Verification items for the finished model (mm, model axes). Face numbers are marked on the shaded views. A direction names the side the tool comes from. Coordinates: 2 decimals unless noted, no trailing zeros. Order: outer loops, then holes, each group sorted by start corner. A loop starts at its lowest first (then second) coordinate and runs counter-clockwise, first axis right, second up.
Q1. Cross-section at C-C, the plane y = 8.5. Record the boundary of the cut face in (x, z), and give its area (3 significant figures).
Q2. Cross-section at A-A, the plane x = 45. Record the boundary of the cut face in (y, z), and give its area (3 significant figures).
Q3. Set-up check for the marked faces 1 and 2: record each of +Z, -Z, +X, -X, +Y, -Y from which the full face is reachable in a straight line by a thin tool's end or side.
Q4. Cross-section at D-D, the plane z = 35. Record the boundary of the cut face in (x, y).
Q5. Depth check by flat-ended pin: P1, Ø8, axis at x = 26.75, z = 8, coming from the +Y side; P2, Ø2.5, axis at x = 37, y = 17, coming from the +Z side. Enter the tip coordinate at first touch or a pass-through.
Q6. Draft check along X on the marked faces 3, 4, 5 and 6. Enter one of: pulls with the +X half, pulls with the -X half, needs draft (parallel to the pull), parting line crosses it, or undercut.
Q7. Thickness scan on line 1 (X direction, y = 21, z = 39); line 2 (Y direction, x = 45, z = 10); line 3 (Y direction, x = 45, z = 31.5). Record the ranges inside material, lowest first.
Q8. Cross-section at B-B, the plane x = 26.75. Record the boundary of the cut face in (y, z).
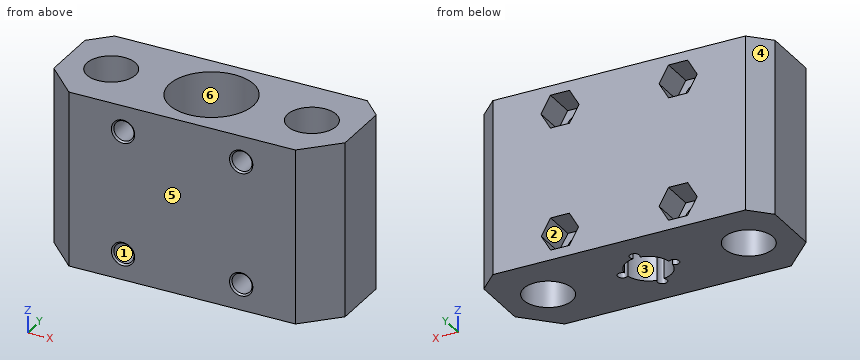
from build123d import *

# Parameters (mm, degrees)
SKETCH1_W           = 90
SKETCH1_H           = 34
SKETCH1_R           = 7
SKETCH1_R_2         = 7.5
BOSS_EXTRUDE1_DEPTH = 54
CHAMFER1_SIZE       = 6
CHAMFER2_SIZE       = 10
SKETCH2_R           = 13
CUT_EXTRUDE1_DEPTH  = 32
SKETCH3_R           = 3.1
CUT_EXTRUDE2_DEPTH  = 111.326787318
CUT_EXTRUDE3_DEPTH  = 10
SKETCH5_R           = 1.5
CUT_EXTRUDE4_DEPTH  = 102.390334845
CIRPATTERN1_COUNT   = 4
CHAMFER3_SIZE       = 0.5


with BuildPart() as part:
    # Sketch1 → Boss-Extrude1 (new body)
    with BuildSketch(Plane.XY):
        with Locations((45, 17)):
            Rectangle(SKETCH1_W, SKETCH1_H)
        with Locations((45, 17)):
            Circle(SKETCH1_R, mode=Mode.SUBTRACT)
        with Locations((14, 17)):
            Circle(SKETCH1_R_2, mode=Mode.SUBTRACT)
        with Locations((76, 17)):
            Circle(SKETCH1_R_2, mode=Mode.SUBTRACT)
    extrude(amount=BOSS_EXTRUDE1_DEPTH)

    # Chamfer1
    chamfer1_edges = [part.edges().sort_by_distance(p)[0] for p in [
        (0, 34, 27),
        (90, 34, 27),
    ]]
    chamfer(chamfer1_edges, length=CHAMFER1_SIZE)

    # Chamfer2
    chamfer2_edges = [part.edges().sort_by_distance(p)[0] for p in [
        (90, 0, 27),
        (0, 0, 27),
    ]]
    chamfer(chamfer2_edges, length=CHAMFER2_SIZE)

    # Sketch2 → Cut-Extrude1 (cut)
    with BuildSketch(Plane.XY.offset(54)):
        with Locations((45, 17)):
            Circle(SKETCH2_R)
    extrude(amount=-CUT_EXTRUDE1_DEPTH, mode=Mode.SUBTRACT)

    # Sketch3 → Cut-Extrude2 (cut, through all)
    with BuildSketch(Plane(origin=(0, 34, 0), x_dir=(1, 0, 0), z_dir=(0, 1, 0))):
        with Locations(Location((26.75, -8, 0), (0, 0, 270))):
            Circle(SKETCH3_R)
        with Locations(Location((63.25, -8, 0), (0, 0, 270))):
            Circle(SKETCH3_R)
        with Locations(Location((63.25, -46, 0), (0, 0, 270))):
            Circle(SKETCH3_R)
        with Locations(Location((26.75, -46, 0), (0, 0, 270))):
            Circle(SKETCH3_R)
    extrude(amount=-CUT_EXTRUDE2_DEPTH, mode=Mode.SUBTRACT)

    # Sketch4 → Cut-Extrude3 (cut)
    with BuildSketch(Plane(origin=(0, 34, 0), x_dir=(1, 0, 0), z_dir=(0, 1, 0))):
        Polygon((23.805513627, -13.1), (29.694486373, -13.1), (32.638972746, -8), (29.694486373, -2.9), (23.805513627, -2.9), (20.861027254, -8), align=None)
        Polygon((60.363248654, -13), (66.136751346, -13), (69.023502692, -8), (66.136751346, -3), (60.363248654, -3), (57.476497308, -8), align=None)
        Polygon((60.305513627, -51.1), (66.194486373, -51.1), (69.138972746, -46), (66.194486373, -40.9), (60.305513627, -40.9), (57.361027254, -46), align=None)
        Polygon((29.694486373, -51.1), (32.638972746, -46), (29.694486373, -40.9), (23.805513627, -40.9), (20.861027254, -46), (23.805513627, -51.1), align=None)
    extrude(amount=-CUT_EXTRUDE3_DEPTH, mode=Mode.SUBTRACT)

    # Sketch5 → Cut-Extrude4 (cut, through all)
    with BuildSketch(Plane.XY.offset(22)):
        with Locations((45, 25)):
            Circle(SKETCH5_R)
    cut_extrude4 = extrude(amount=-CUT_EXTRUDE4_DEPTH, mode=Mode.SUBTRACT)

    # CirPattern1: Cut-Extrude4 ×4 about axis
    cirpattern1_axis = Axis((45, 17, 0), (0, 0, 1))
    for i in range(1, CIRPATTERN1_COUNT):
        add(cut_extrude4.rotate(cirpattern1_axis, i * 360 / CIRPATTERN1_COUNT), mode=Mode.SUBTRACT)

    # Chamfer3
    chamfer3_edges = [part.edges().sort_by_distance(p)[0] for p in [
        (26.75, 0, 42.9),
        (63.25, 0, 42.9),
        (63.25, 0, 4.9),
        (26.75, 0, 4.9),
    ]]
    chamfer(chamfer3_edges, length=CHAMFER3_SIZE)


solid = part.part
Check values:
1. outline: (1.5, 0) - (43.59, 0) - (43.59, 22) - (35.16, 22) - (35.16, 54) - (1.5, 54) - close; (46.41, 0) - (88.5, 0) - (88.5, 54) - (54.84, 54) - (54.84, 22) - (46.41, 22) - close; hole circle Ø6.2 at (26.75, 8); hole circle Ø6.2 at (26.75, 46); hole circle Ø6.2 at (63.25, 8); hole circle Ø6.2 at (63.25, 46)
1. area: 3,890 mm2
2. outline: (0, 0) - (7.5, 0) - (7.5, 22) - (4, 22) - (4, 54) - (0, 54) - close; (26.5, 0) - (34, 0) - (34, 54) - (30, 54) - (30, 22) - (26.5, 22) - close
2. area: 586 mm2
3. face 1: +Y, -Y
3. face 2: +Y
4. outline: (0, 10) - (10, 0) - (80, 0) - (90, 10) - (90, 28) - (84, 34) - (6, 34) - (0, 28) - close; hole circle Ø15 at (14, 17); hole circle Ø26 at (45, 17); hole circle Ø15 at (76, 17)
5. P1: stops at y = 24
5. P2: passes through
6. face 3: undercut
6. face 4: pulls with the -X half
6. face 5: needs draft
6. face 6: undercut
7. line 1: x = 0 to 7.66, 20.34 to 32.63, 57.37 to 69.66, 82.34 to 90
7. line 2: y = 0 to 7.5, 26.5 to 34
7. line 3: y = 0 to 4, 30 to 34
8. outline: (0, 0) - (34, 0) - (34, 2.9) - (24, 2.9) - (24, 4.9) - (0.5, 4.9) - (0, 4.4) - close; (0, 11.6) - (0.5, 11.1) - (24, 11.1) - (24, 13.1) - (34, 13.1) - (34, 40.9) - (24, 40.9) - (24, 42.9) - (0.5, 42.9) - (0, 42.4) - close; (0, 49.6) - (0.5, 49.1) - (24, 49.1) - (24, 51.1) - (34, 51.1) - (34, 54) - (0, 54) - close
